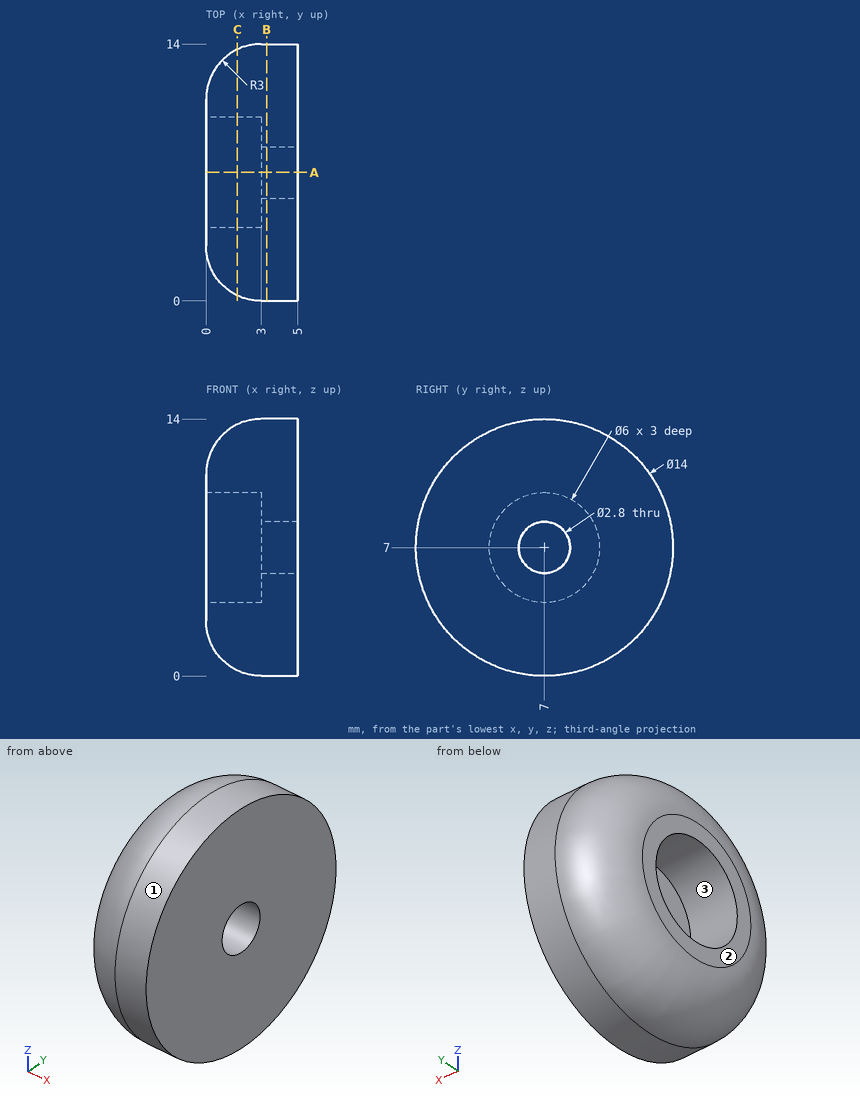
Geometry check sheet. Reference: drawing and pictorial views, mm from the part's lowest x, y, z. Round coordinates to 2 decimals unless told otherwise and drop trailing zeros. Write each loop counter-clockwise with the first axis right and the second up, starting at its lowest first coordinate (ties: lowest second). Pieces come first, ordered by that corner, then holes.
1. Draft check along Z on the marked faces 1, 2 and 3. Enter one of: +Z half, -Z half, draft (parallel to the pull), parting line (faces both ways), or undercut.
2. Section check A-A on y = 7. Enter the section's corners in (x, z).
3. Scan lines: L1, parallel to Y at x = 3.5, z = 7; L2, parallel to Y at x = 0.65, z = 8.75; L3, parallel to Z at x = 0.65, y = 7.75. Record each from-to range of solid material in increasing order.
4. Section check B-B on x = 3.3. Enter the section's corners in (y, z), plus the area to 3 significant figures.
5. Section check C-C on x = 1.7. Enter the section's corners in (y, z), plus the area to 3 significant figures.
6. Gauge pin test, flat ends, axial feed: P1, Ø1.5, axis at x = 2, y = 4.5, coming from the -Z side; P2, Ø3, axis at y = 7, z = 7, coming from the +X side; P3, Ø1, axis at x = 3, z = 4.5, coming from the +Y side; P4, Ø1, axis at x = 2, y = 8, coming from the -Z side. Record the tip position at first contact, or that the pin passes through.
Answer:
1. face 1: parting line
1. face 2: draft
1. face 3: undercut
2. outline: (0, 3) arc R3 ccw to (3, 0) - (5, 0) - (5, 5.6) - (3, 5.6) - (3, 4) - (0, 4) - close; (0, 10) - (3, 10) - (3, 8.4) - (5, 8.4) - (5, 14) - (3, 14) arc R3 ccw to (0, 11) - close
3. L1: y = 0 to 5.6, 8.4 to 14
3. L2: y = 1.4 to 4.56, 9.44 to 12.6
3. L3: z = 1.18 to 4.1, 9.9 to 12.82
4. outline: circle Ø14 at (7, 7); hole circle Ø2.8 at (7, 7)
4. area: 148 mm2
5. outline: circle Ø13.41 at (7, 7); hole circle Ø6 at (7, 7)
5. area: 113 mm2
6. P1: stops at z = 0.32
6. P2: stops at x = 5
6. P3: stops at y = 13.71
6. P4: stops at z = 0.09
